from build123d import *

# Parameters (mm, degrees)
F1_DEPTH = 18.2
F3_DEPTH = 6.5
F4_R     = 4
F5_DEPTH = 12.5
F6_R     = 3


with BuildPart() as f1:
    # F0 (on Top) → F1 (new body)
    with BuildSketch(Plane.XY):
        Polygon((4.474465, -7.75), (8.948929, 0), (4.474465, 7.75), (-4.474465, 7.75), (-8.948929, 0), (-4.474465, -7.75), align=None)
    extrude(amount=F1_DEPTH)

    # F2 (on Top) → F3 (cut)
    with BuildSketch(Plane.XY):
        Polygon((3.608439, -6.25), (7.216878, 0), (3.608439, 6.25), (-3.608439, 6.25), (-7.216878, 0), (-3.608439, -6.25), align=None)
    extrude(amount=F3_DEPTH, mode=Mode.SUBTRACT)

    # F4 (on Top) → F5 (cut)
    with BuildSketch(Plane.XY):
        Circle(F4_R)
    extrude(amount=F5_DEPTH, mode=Mode.SUBTRACT)

    # F6
    f6_edges = [f1.edges().sort_by_distance(p)[0] for p in [
        (8.948929, 0, 9.1),
        (4.474465, -7.75, 9.1),
        (-4.474465, -7.75, 9.1),
    ]]
    fillet(f6_edges, radius=F6_R)


solid = f1.part
Geometry: final body of the model. Coordinates: model frame, mm. A direction names the side the tool comes from. Give positions to 0.01 mm unless a question says otherwise; leave off trailing zeros. Write each loop counter-clockwise with the first axis right and the second up, starting at its lowest first coordinate (ties: lowest second). Pieces come first, ordered by that corner, then holes. Notation, with made-up numbers: (63, 3.5) -> (75, 3.5) arc R19 cw to (75, 35.5) -> close; hole circle Ø7 at (12.5, -26.5). An arc over 180 degrees is marked (long way). Answer as a JSON object with one key per item and string values.
1. Cut plane A-A on z = 4.5. Output: boundary loops of the cut face in (x, y), and give its area (3 significant figures).
Ans:
{"outline": "(-8.95, 0) -> (-5.34, -6.25) arc R3 ccw to (-2.74, -7.75) -> (2.74, -7.75) arc R3 ccw to (5.34, -6.25) -> (8.08, -1.5) arc R3 ccw to (8.08, 1.5) -> (4.47, 7.75) -> (-4.47, 7.75) -> close; hole (-7.22, 0) -> (-3.61, -6.25) -> (3.61, -6.25) -> (7.22, 0) -> (3.61, 6.25) -> (-3.61, 6.25) -> close", "area": "71.3 mm^2"}
2. Cut plane C-C on y = 0.25. Output: boundary loops of the cut face in (x, z), and give its area (3 significant figures).
Ans:
{"outline": "(-8.8, 0) -> (-7.07, 0) -> (-7.07, 6.5) -> (-3.99, 6.5) -> (-3.99, 12.5) -> (3.99, 12.5) -> (3.99, 6.5) -> (7.07, 6.5) -> (7.07, 0) -> (8.47, 0) -> (8.47, 18.2) -> (-8.8, 18.2) -> close", "area": "175 mm^2"}
3. Cut plane D-D on z = 7.25. Output: boundary loops of the cut face in (x, y).
Ans:
{"outline": "(-8.95, 0) -> (-5.34, -6.25) arc R3 ccw to (-2.74, -7.75) -> (2.74, -7.75) arc R3 ccw to (5.34, -6.25) -> (8.08, -1.5) arc R3 ccw to (8.08, 1.5) -> (4.47, 7.75) -> (-4.47, 7.75) -> close; hole circle Ø8 at (0, 0)"}
4. Ray query, probe 1 along Y at (x, z) = (0.75, 5); probe 2 along Y at (x, z) = (0, 11.2); probe 3 along X at (y, z) = (-2, 8). Return the intervals inside material, ascending. Write a range as from..to.
Ans:
{"probe 1": "y = -7.75..-6.25, 6.25..7.75", "probe 2": "y = -7.75..-4, 4..7.75", "probe 3": "x = -7.79..-3.46, 3.46..7.79"}
5. Access query for faces 1 (the flat face through (-6.68, 3.93, 8.97)), 2 (the flat face through (3, 3, 6.5)). Directions: +Z, -Z, +X, -X, +Y, -Y. A direction counts if a zero-diameter tool reaches every point of the face in a straight line with its end or side. Return the directions, or none.
Ans:
{"face 1": "+Z, -Z, -X, +Y", "face 2": "-Z"}
6. Contact query for flat-ended pins moving along their axis: pin 1 (1 mm diameter, centred on y = -6, z = 15.5, fed in from +X); pin 2 (4 mm diameter, centred on y = -4, z = 6, fed in from -X); pin 3 (4 mm diameter, centred on x = -1, y = 2, fed in from -Z). Output: stop coordinate, or through.
Ans:
{"pin 1": "stops at x = 5.77", "pin 2": "stops at x = -7.79", "pin 3": "stops at z = 6.5"}
7. Cut plane B-B on x = 0. Output: boundary loops of the cut face in (y, z), and give its area (3 significant figures).
Ans:
{"outline": "(-7.75, 0) -> (-6.25, 0) -> (-6.25, 6.5) -> (-4, 6.5) -> (-4, 12.5) -> (4, 12.5) -> (4, 6.5) -> (6.25, 6.5) -> (6.25, 0) -> (7.75, 0) -> (7.75, 18.2) -> (-7.75, 18.2) -> close", "area": "153 mm^2"}
8. Mould query, pull axis X, two halves, no side actions, for faces 3 (the flat face through (5.387, -3.169, 3.204)), 4 (the flat face through (-5.387, 3.169, 3.204)), 5 (the cylindrical face through (8.485, -0.022, 9.227)), 6 (the flat face through (0, -7.75, 9)). Classes: pulls with the +X half, pulls with the -X half, needs draft (parallel to the pull), parting line crosses it, or undercut.
Ans:
{"face 3": "undercut", "face 4": "undercut", "face 5": "pulls with the +X half", "face 6": "needs draft"}
